Input: dimensioned drawing with shaded views. Units: mm. Origin: part minimum x, y, z. Coordinates: 2 decimals unless noted, no trailing zeros. Order: outer loops, then holes, each group sorted by start corner. A loop starts at its lowest first (then second) coordinate and runs counter-clockwise, first axis right, second up. Notation, with made-up numbers: (-20, -39.5) -> (18, -39.5) arc R15 cw to (18, -19.5) -> close; hole circle Ø9 at (2.5, 23). An arc over 180 degrees is marked (long way). Answer in a Markdown table with one row per item. Add a question column.
1) Section query C-C on z = 8.5. Count the separate pieces of the cut face and the enclosed holes in it, then the cut area to 3 significant figures.
2) Contact query for flat-ended pins moving along their axis: P1, Ø6, axis at x = 5, z = 3.5, coming from the +Y side; P2, Ø6, axis at x = 40, z = 11.5, coming from the -Y side; P3, Ø10, axis at y = 18, z = 7.5, coming from the -X side. Output: stop coordinate, or through.
3) Section query D-D on y = 33.5. Return the cut outline in (x, z), then the cut area to 3 significant figures.
4) Pull-direction query (Y, two-part tool) for the marked faces 1, 2 and 3; classes: +Y half, -Y half, draft (parallel to the pull), parting line (faces both ways), or undercut.
5) Section query A-A on x = 24.5. Return the cut outline in (y, z).
6) Ray query, line 1 (Y direction, x = 25, z = 5.25); line 2 (Y direction, x = 23, z = 9.5); line 3 (Z direction, x = 27.5, y = 32.5). Return the intervals inside material, ascending. Write a range as from..to.
7) Section query B-B on y = 10.5. Return the cut outline in (x, z), then the cut area to 3 significant figures.
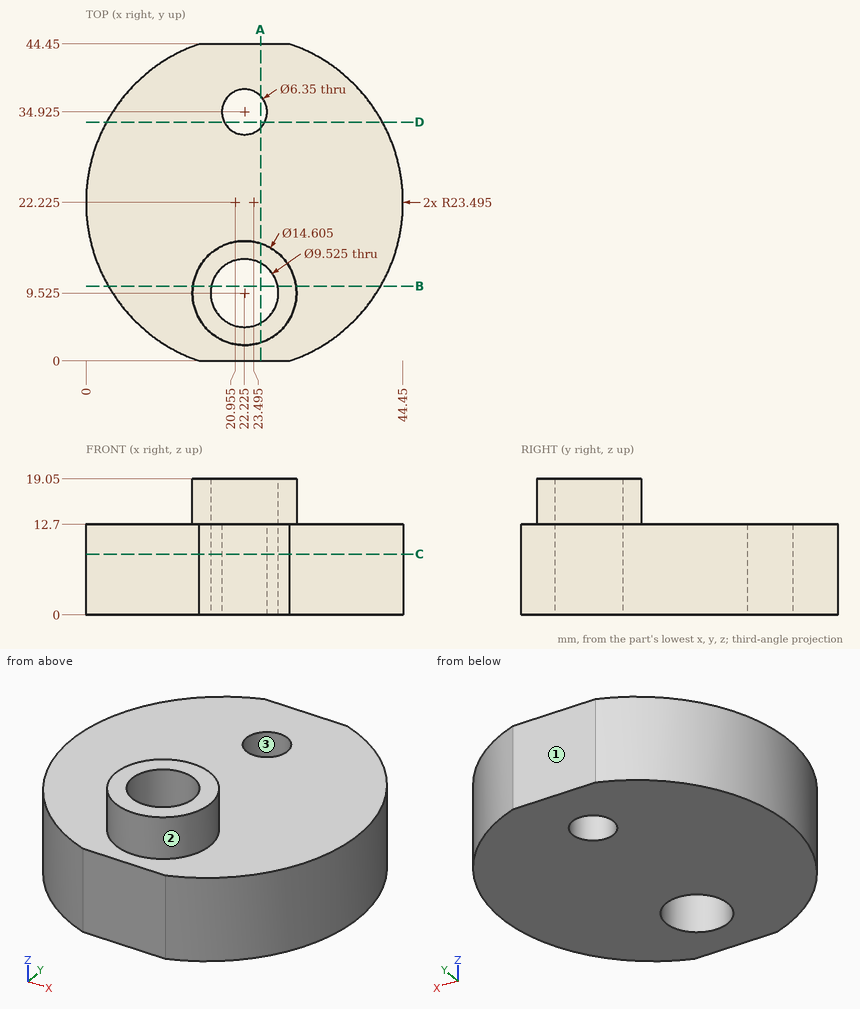
Result:
| question | item | result |
|---|---|---|
| 1 | separate pieces | 1 |
| 1 | enclosed holes | 2 |
| 1 | area | 1,490 mm2 |
| 2 | P1 | y = 39.89 |
| 2 | P2 | y = 5.06 |
| 2 | P3 | x = 0 |
| 3 | outline | (2.88, 0) -> (19.39, 0) -> (19.39, 12.7) -> (2.88, 12.7) -> close; (25.06, 0) -> (41.57, 0) -> (41.57, 12.7) -> (25.06, 12.7) -> close |
| 3 | area | 419 mm2 |
| 4 | face 1 | +Y half |
| 4 | face 2 | parting line |
| 4 | face 3 | undercut |
| 5 | outline | (0, 0) -> (5.34, 0) -> (5.34, 19.05) -> (2.59, 19.05) -> (2.59, 12.7) -> (0, 12.7) -> close; (13.71, 0) -> (32.71, 0) -> (32.71, 12.7) -> (16.46, 12.7) -> (16.46, 19.05) -> (13.71, 19.05) -> close; (37.14, 0) -> (44.45, 0) -> (44.45, 12.7) -> (37.14, 12.7) -> close |
| 6 | line 1 | 0..5.65, 13.4..33.38, 36.47..44.45 |
| 6 | line 2 | 0..4.83, 14.22..31.85, 38..44.45 |
| 6 | line 3 | 0..12.7 |
| 7 | outline | (3.13, 0) -> (17.56, 0) -> (17.56, 19.05) -> (14.99, 19.05) -> (14.99, 12.7) -> (3.13, 12.7) -> close; (26.89, 0) -> (41.32, 0) -> (41.32, 12.7) -> (29.46, 12.7) -> (29.46, 19.05) -> (26.89, 19.05) -> close |
| 7 | area | 399 mm2 |
